from build123d import *

# Parameters (mm, degrees)
F0_W     = 50
F0_H     = 50
F1_DEPTH = 25
F2_R     = 15
F3_R     = 15
F4_R     = 15
F5_R     = 15
F6_R     = 15
F7_T     = 2.5


# Not quite as in the source:
# - a shell that OpenCascade refuses in one call is made with other operations: the cavity is built on its own and cut out


with BuildPart() as f1:
    # F0 (on Top) → F1 (new body, symmetric)
    with BuildSketch(Plane.XY):
        Rectangle(F0_W, F0_H)
    extrude(amount=F1_DEPTH, both=True)

    # F2
    f2_edges = [f1.edges().sort_by_distance(p)[0] for p in [
        (-25, 0, 25),
    ]]
    fillet(f2_edges, radius=F2_R)

    # F3
    f3_edges = [f1.edges().sort_by_distance(p)[0] for p in [
        (7.5, -25, 25),
    ]]
    fillet(f3_edges, radius=F3_R)

    # F4
    f4_edges = [f1.edges().sort_by_distance(p)[0] for p in [
        (25, 7.5, 25),
    ]]
    fillet(f4_edges, radius=F4_R)

    # F5
    f5_edges = [f1.edges().sort_by_distance(p)[0] for p in [
        (0, 25, 25),
    ]]
    fillet(f5_edges, radius=F5_R)

    # F6
    f6_edges = [f1.edges().sort_by_distance(p)[0] for p in [
        (25, 0, -25),
    ]]
    fillet(f6_edges, radius=F6_R)

    # F7: shell of thickness 2.5, made by hand


with BuildPart() as f7_core1:
    # F7_t2: copy of F1
    add(f1.part)

    # the walls: a layer under each face that stays
    f7_faces = [f7_core1.faces().sort_by_distance(p)[0] for p in [
        (0, 0, -25),
        (20.6066017178, 0, -20.6066017178),
        (0, -20.6066017178, -20.6066017178),
        (0, 20.6066017178, -20.6066017178),
        (-20.6066017178, 0, -20.6066017178),
        (17.5, -17.5, -20.6066017178),
        (25, 0, 0),
        (17.5, 17.5, -20.6066017178),
        (-17.5, -17.5, -20.6066017178),
        (0, -25, 0),
        (0, 25, 0),
        (-17.5, 17.5, -20.6066017178),
        (-25, 0, 0),
        (20.6066017178, -20.6066017178, 0),
        (20.6066017178, 20.6066017178, 0),
        (-20.6066017178, -20.6066017178, 0),
        (-20.6066017178, 20.6066017178, 0),
        (20.6066017178, -17.5, 17.5),
        (17.5, 20.6066017178, 17.5),
        (-17.5, -20.6066017178, 17.5),
        (-17.5, 20.6066017178, 17.5),
    ]]
    thicken(f7_faces, amount=-F7_T, mode=Mode.SUBTRACT)


with BuildPart() as f1_1:
    add(f1.part)

    # what is left inside the walls is the cavity
    f7_cavity = [f7_core1.part.solids().sort_by_distance(p)[0] for p in [
        (3.333333, 20.588924, 20.588924),
    ]]
    add(f7_cavity, mode=Mode.SUBTRACT)


solid = f1_1.part
Geometry: final body of the model. Coordinates: model frame, mm. A direction names the side the tool comes from. Coordinates: 2 decimals unless noted, no trailing zeros. Order: outer loops, then holes, each group sorted by start corner. A loop starts at its lowest first (then second) coordinate and runs counter-clockwise, first axis right, second up.
1) Section B-B (y = -0.5). Return loops of the section in (x, z), then the cut area to 3 significant figures.
Result sheet:
outline: (-25, -10) arc R15 ccw to (-10, -25) - (10, -25) arc R15 ccw to (25, -10) - (25, 10) - (22.5, 10) - (22.5, -10) arc R12.5 cw to (10, -22.5) - (-10, -22.5) arc R12.5 cw to (-22.5, -10) - (-22.5, 10) - (-25, 10) - close
area: 258 mm2
2) Set-up query: faces 1 (the flat face through (19, -10, 19)), 2 (the flat face through (0, 22.5, 0)), 3 (the flat face through (10, -19, 19)). Return all of +Z, -Z, +X, -X, +Y, -Y with unobstructed straight access to the full face (end or side cutting, diameter ignored); none if empty.
Result sheet:
face 1: +Z, +X, -X
face 2: +Z
face 3: +Z, +Y, -Y
3) Ray query, probe 1 along Y at (x, z) = (-6.5, -5); probe 2 along Z at (x, y) = (9.5, 1.5); probe 3 along X at (y, z) = (-10.5, 21). Return the intervals inside material, ascending.
Result sheet:
probe 1: y = -25 to -22.5, 22.5 to 25
probe 2: z = -25 to -22.5
probe 3: x = -20.19 to -15.92, 15.92 to 20.19
4) Section A-A (z = 5). Return loops of the section in (x, y).
Result sheet:
outline: (-25, -10) arc R15 ccw to (-10, -25) - (10, -25) arc R15 ccw to (25, -10) - (25, 10) arc R15 ccw to (10, 25) - (-10, 25) arc R15 ccw to (-25, 10) - close; hole (-22.5, -10) arc R12.5 ccw to (-10, -22.5) - (10, -22.5) arc R12.5 ccw to (22.5, -10) - (22.5, 10) arc R12.5 ccw to (10, 22.5) - (-10, 22.5) arc R12.5 ccw to (-22.5, 10) - close
5) Draft query along Z for faces 4 (the cylindrical face through (0.14, -20.49, -20.72)), 5 (the cylindrical face through (0.14, -18.741, -18.935)), 6 (the flat face through (10, 19, 19)), 7 (the cylindrical face through (18.741, -18.935, 0.14)). Return one class per face: released by +Z, released by -Z, zero draft, split by the parting line, or undercut.
Result sheet:
face 4: released by -Z
face 5: released by +Z
face 6: zero draft
face 7: undercut
6) First-contact query: P1, Ø2, axis at x = 19.5, z = 9, coming from the -Y side; P2, Ø10, axis at y = 2, z = -16, coming from the +X side; P3, Ø0.8, axis at x = 24, y = 3.5, coming from the +Z side. Flat tips, straight axial feed; report the tip coordinate or a pass-through.
Result sheet:
P1: stops at y = -22.36
P2: stops at x = 24.97
P3: stops at z = 10
7) Section D-D (z = 15). Return loops of the section in (x, y), then the cut area to 3 significant figures.
Result sheet:
outline: (-24.14, -10) arc R14.14 ccw to (-10, -24.14) - (-10, -21.46) arc R11.46 cw to (-21.46, -10) - close; (-24.14, 10) - (-21.46, 10) arc R11.46 cw to (-10, 21.46) - (-10, 24.14) arc R14.14 ccw to start; (10, -24.14) arc R14.14 ccw to (24.14, -10) - (21.46, -10) arc R11.46 cw to (10, -21.46) - close; (10, 21.46) arc R11.46 cw to (21.46, 10) - (24.14, 10) arc R14.14 ccw to (10, 24.14) - close
area: 216 mm2
